Check sheet for the drawn part. Datum: minimum x, y, z corner. Units: mm. A direction names the side the tool comes from. Round coordinates to 2 decimals unless told otherwise and drop trailing zeros. Write each loop counter-clockwise with the first axis right and the second up, starting at its lowest first coordinate (ties: lowest second). Pieces come first, ordered by that corner, then holes.
Item 1: Material ranges on line 1 (Z direction, x = 4.5, y = 1); line 2 (X direction, y = 0.55, z = 24.5); line 3 (Z direction, x = 4.5, y = 0.9), recorded low to high.
Item 2: Go/stop test with flat-tipped pins: pin 1 Ø4 at (x, z) = (4.5, 8.5) entering from +Y; pin 2 Ø3 at (x, y) = (15.5, 11) entering from +Z; pin 3 Ø1.5 at (x, y) = (5, 4) entering from +Z. Record where each tip stops, or that it passes through.
Item 3: Cross-section at A-A on y = 8.2. Enter the section's corners in (x, z).
Item 4: Cross-section at D-D on x = 12.5. Enter the section's corners in (y, z).
Item 5: Release check for a two-part mould opening along Y. For the marked faces 1, 2 and 3 record: +Y half, -Y half, draft (parallel to the pull), parting line (faces both ways), or undercut.
Item 6: Cross-section at B-B on z = 8.5. Enter the section's corners in (x, y), plus the area to 3 significant figures.
Item 7: Tool access check on the marked faces 4 and 5. Record the directions out of +Z, -Z, +X, -X, +Y, -Y that give a thin tool (end or side, any length) a straight path to the whole face; none if there is none.
Item 8: Cross-section at C-C on x = 20.5. Enter the section's corners in (y, z), plus the area to 3 significant figures.
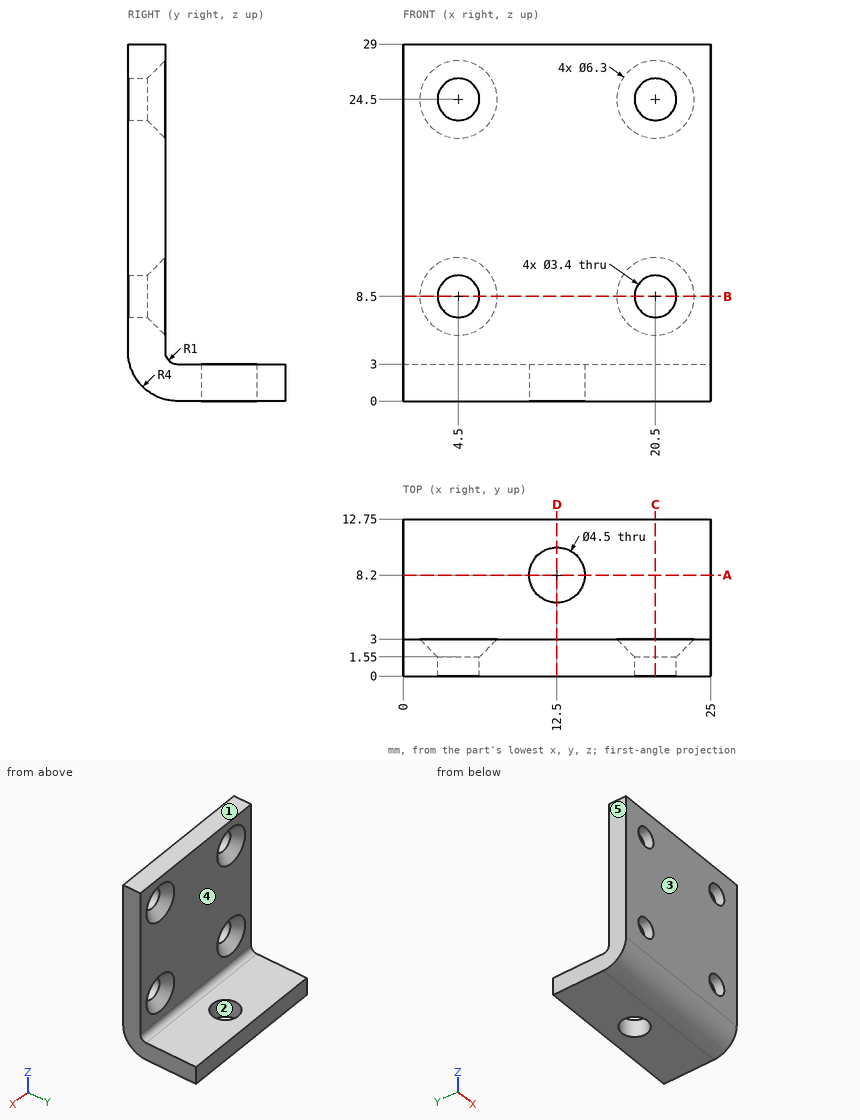
Response values:
1. line 1: z = 1.35 to 6.8, 10.2 to 22.8, 26.2 to 29
1. line 2: x = 0 to 2.8, 6.2 to 18.8, 22.2 to 25
1. line 3: z = 1.47 to 6.8, 10.2 to 22.8, 26.2 to 29
2. pin 1: stops at y = 1.85
2. pin 2: stops at z = 3
2. pin 3: stops at z = 3.34
3. outline: (0, 0) - (10.25, 0) - (10.25, 3) - (0, 3) - close; (14.75, 0) - (25, 0) - (25, 3) - (14.75, 3) - close
4. outline: (0, 4) arc R4 ccw to (4, 0) - (5.95, 0) - (5.95, 3) - (4, 3) arc R1 cw to (3, 4) - (3, 29) - (0, 29) - close; (10.45, 0) - (12.75, 0) - (12.75, 3) - (10.45, 3) - close
5. face 1: draft
5. face 2: undercut
5. face 3: -Y half
6. outline: (0, 0) - (2.8, 0) - (2.8, 1.55) - (1.35, 3) - (0, 3) - close; (6.2, 0) - (18.8, 0) - (18.8, 1.55) - (17.35, 3) - (7.65, 3) - (6.2, 1.55) - close; (22.2, 0) - (25, 0) - (25, 3) - (23.65, 3) - (22.2, 1.55) - close
6. area: 50.4 mm2
7. face 4: +Z, +X, -X, +Y
7. face 5: +Z, -Z, -X, +Y, -Y
8. outline: (0, 4) arc R4 ccw to (4, 0) - (12.75, 0) - (12.75, 3) - (4, 3) arc R1 cw to (3, 4) - (3, 5.35) - (1.55, 6.8) - (0, 6.8) - close; (0, 10.2) - (1.55, 10.2) - (3, 11.65) - (3, 21.35) - (1.55, 22.8) - (0, 22.8) - close; (0, 26.2) - (1.55, 26.2) - (3, 27.65) - (3, 29) - (0, 29) - close
8. area: 88.4 mm2
